Could you check a few things on this model? Use its own coordinates, in mm. A direction names the side the tool comes from. Coordinates: 2 decimals unless noted, no trailing zeros. Write each loop counter-clockwise with the first axis right and the second up, starting at its lowest first coordinate (ties: lowest second). Pieces come first, ordered by that corner, then holes.
Item 1: If I drill on probe 1 along Z at (x, y) = (17, 7.5); probe 2 along Z at (x, y) = (30, 0.45), over which ranges is the centre line in solid material (lowest first)?
Item 2: Which directions (+Z, -Z, +X, -X, +Y, -Y) give clear straight access to the entire face, cutting with the end or side of a thin tool? Please do faces 1 (the flat face through (1, 21, 1.473)), 2 (the flat face through (1, 20, 0)).
Item 3: Thinking about a two-plate mould opening in X: for faces 3 (the cylindrical face through (-30.54, 7.56, 0.73)), 4 (the flat face through (-40, 1, 11)), 5 (the flat face through (1, 0, 21)), which applies, +X half, -X half, draft (parallel to the pull), parting line (faces both ways), or undercut?
Item 4: For P1, Ø2, axis at x = -25, z = 15.5, coming from the +Y side; P2, Ø10, axis at x = 8.5, y = 25, coming from the +Z side, each with a flat end and sliding along its axis, tell me the tip position at first contact or that it passes through.
Item 5: I want a section at D-D on x = -29. Please give me the cut outline in (y, z), then the cut area to 3 significant figures.
Item 6: I want a section at B-B on z = 18.75. Please give me the cut outline in (x, y).
Item 7: I want a section at C-C on y = 29. Please give me the cut outline in (x, z).
Item 8: I want a section at A-A on x = 30. Please give me the cut outline in (y, z), then the cut area to 3 significant figures.
from build123d import *

# Parameters (mm, degrees)
F1_DEPTH = 40
F2_R     = 2.5
F3_DEPTH = 12.7
F4_R     = 2.5
F5_DEPTH = 12.7


with BuildPart() as f1:
    # F0 (on Right) → F1 (new body, symmetric)
    with BuildSketch(Plane.YZ):
        with BuildLine():
            Line((1.4732, 38.1), (0, 38.1))
            Line((0, 38.1), (0, 2.54))
            ThreePointArc((0, 2.54), (0.7439487758, 0.7439487758), (2.54, 0))
            Line((2.54, 0), (38.1, 0))
            Line((38.1, 0), (38.1, 1.4732))
            Line((38.1, 1.4732), (4.0132, 1.4732))
            ThreePointArc((4.0132, 1.4732), (2.2171487758, 2.2171487758), (1.4732, 4.0132))
            Line((1.4732, 4.0132), (1.4732, 38.1))
        make_face()
    extrude(amount=F1_DEPTH, both=True)

    # F2 (on Top) → F3 (cut, symmetric)
    with BuildSketch(Plane.XY):
        with Locations((-30, 10)):
            Circle(F2_R)
        with Locations((0, 10)):
            Circle(F2_R)
        with Locations((30, 10)):
            Circle(F2_R)
    extrude(amount=F3_DEPTH, both=True, mode=Mode.SUBTRACT)

    # F4 (on Front) → F5 (cut, symmetric)
    with BuildSketch(Plane.XZ):
        with Locations((-30, 28.75)):
            Circle(F4_R)
        with Locations((30, 28.75)):
            Circle(F4_R)
        with Locations((20, 18.75)):
            Circle(F4_R)
        with Locations((-20, 18.75)):
            Circle(F4_R)
    extrude(amount=F5_DEPTH, both=True, mode=Mode.SUBTRACT)


solid = f1.part
Response values:
1. probe 1: z = 0 to 1.47
1. probe 2: z = 1.1 to 26.25, 31.25 to 38.1
2. face 1: +Z, +X, -X, +Y
2. face 2: -Z, +X, -X, +Y, -Y
3. face 3: undercut
3. face 4: -X half
3. face 5: draft
4. P1: stops at y = 1.47
4. P2: stops at z = 1.47
5. outline: (0, 2.54) arc R2.54 ccw to (2.54, 0) - (7.71, 0) - (7.71, 1.47) - (4.01, 1.47) arc R2.54 cw to (1.47, 4.01) - (1.47, 26.46) - (0, 26.46) - close; (0, 31.04) - (1.47, 31.04) - (1.47, 38.1) - (0, 38.1) - close; (12.29, 0) - (38.1, 0) - (38.1, 1.47) - (12.29, 1.47) - close
5. area: 96.6 mm2
6. outline: (-40, 0) - (-22.5, 0) - (-22.5, 1.47) - (-40, 1.47) - close; (-17.5, 0) - (17.5, 0) - (17.5, 1.47) - (-17.5, 1.47) - close; (22.5, 0) - (40, 0) - (40, 1.47) - (22.5, 1.47) - close
7. outline: (-40, 0) - (40, 0) - (40, 1.47) - (-40, 1.47) - close
8. outline: (0, 2.54) arc R2.54 ccw to (2.54, 0) - (7.5, 0) - (7.5, 1.47) - (4.01, 1.47) arc R2.54 cw to (1.47, 4.01) - (1.47, 26.25) - (0, 26.25) - close; (0, 31.25) - (1.47, 31.25) - (1.47, 38.1) - (0, 38.1) - close; (12.5, 0) - (38.1, 0) - (38.1, 1.47) - (12.5, 1.47) - close
8. area: 95.4 mm2
